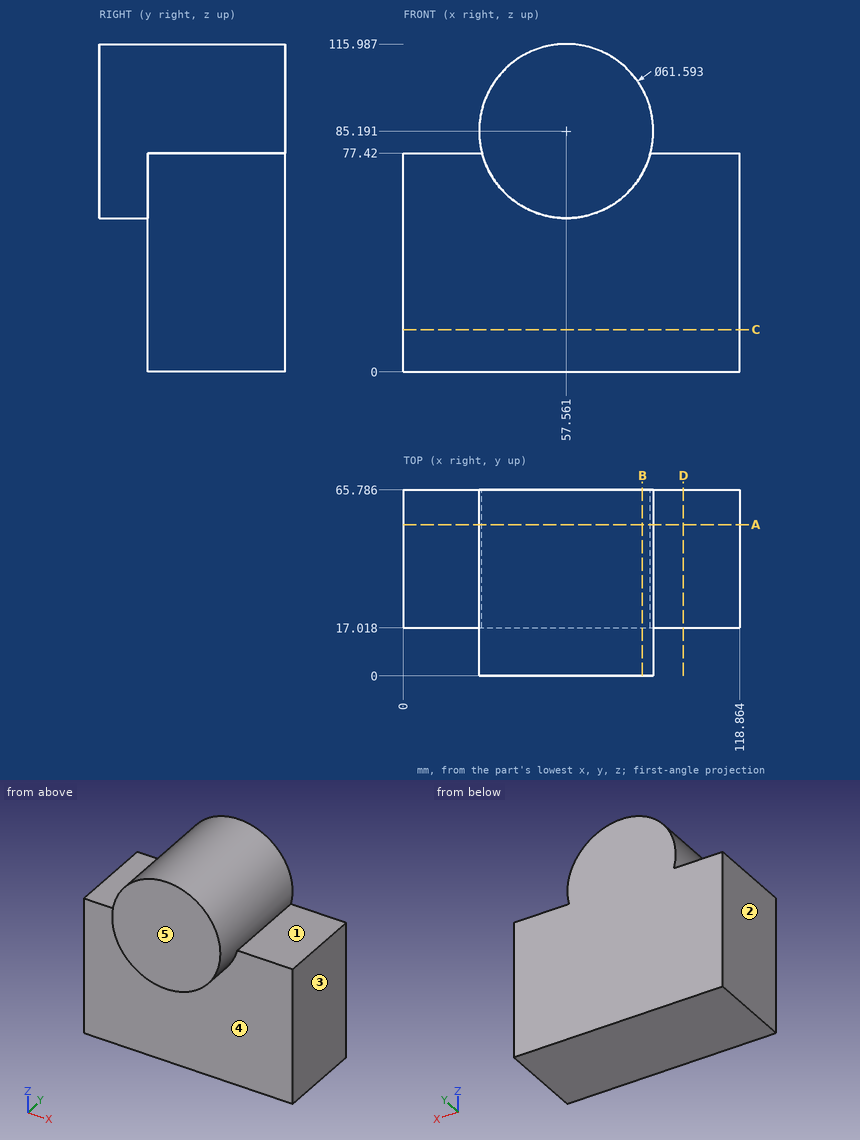
Could you check a few things on this drawing? It's one solid part, dimensions in mm from its lowest x, y, z. A direction names the side the tool comes from. Give positions to 0.01 mm unless a question says otherwise; leave off trailing zeros. Loops run counter-clockwise (first coordinate to the right, second up) from the corner with the lowest first, then second, coordinate; pieces in that order, holes last. Notation, with made-up numbers: M 48,3.25 L 87,3.25 A27 cw 87,35.25 Z; hole C 1,53.5 d6. An arc over 180 degrees is marked long. Return JSON: item names as keys, results as strings.
Item 1: I'm going to push flat-ended pins straight in: pin 1 Ø8 at (y, z) = (37.5, 101.5) entering from -X; pin 2 Ø5 at (x, y) = (51, 8) entering from +Z; pin 3 Ø4 at (x, y) = (23, 36) entering from +Z. Where does each tip first touch, or does it pass through?
A:
{"pin 1": "stops at x = 29.33", "pin 2": "stops at z = 115.72", "pin 3": "stops at z = 77.42"}
Item 2: Thinking about a two-plate mould opening in X: for the marked faces 1, 2 and 3, which applies, released by +X, released by -X, zero draft, split by the parting line, or undercut?
A:
{"face 1": "zero draft", "face 2": "released by -X", "face 3": "released by +X"}
Item 3: Please list where these lines run through material, in increasing order: line 1 (Y direction, x = 50, z = 55) (1 decimal); line 2 (Z direction, x = 11.5, y = 41); line 3 (Z direction, x = 43.5, y = 53).
A:
{"line 1": "y = 17 to 65.8", "line 2": "z = 0 to 77.42", "line 3": "z = 0 to 112.59"}
Item 4: Imagine slicing it at A-A on y = 53.5. List the corners of the cut face in (x, z) for me.
A:
{"outline": "M 0,0 L 118.86,0 L 118.86,77.42 L 87.36,77.42 A30.8 ccw long 27.76,77.42 L 0,77.42 Z"}
Item 5: Imagine slicing it at D-D on x = 99. List the corners of the cut face in (y, z) for me (1 decimal).
A:
{"outline": "M 17,0 L 65.8,0 L 65.8,77.4 L 17,77.4 Z"}
Item 6: On a 3-axis mill with a long thin cutter (end or side, diameter ignored), from which of +Z, -Z, +X, -X, +Y, -Y can I reach the whole of each face in a straight line? I mean the marked faces 4 and 5. Say none if no direction works.
A:
{"face 4": "-Z, -Y", "face 5": "+Z, -Z, +X, -X, -Y"}
Item 7: Imagine slicing it at C-C on z = 15. List the corners of the cut face in (x, y) for me (1 decimal).
A:
{"outline": "M 0,17 L 118.9,17 L 118.9,65.8 L 0,65.8 Z"}
Item 8: Imagine slicing it at B-B on x = 84.5. List the corners of the cut face in (y, z) for me (1 decimal).
A:
{"outline": "M 0,70.3 L 17,70.3 L 17,0 L 65.8,0 L 65.8,100.1 L 0,100.1 Z"}
